Geometry: final body of the model. Coordinates: model frame, mm. A direction names the side the tool comes from. Round coordinates to 2 decimals unless told otherwise and drop trailing zeros. Loops run counter-clockwise (first coordinate to the right, second up) from the corner with the lowest first, then second, coordinate; pieces in that order, holes last. Notation, with made-up numbers: M -3.75,51 L 2.25,51 A28 ccw 2.25,83 Z; hole C -28.5,56 d7. An arc over 180 degrees is marked long. Answer as a JSON object with one key per item and string values.
from build123d import *

# Parameters (mm, degrees)
SKETCH1_W           = 60
SKETCH1_H           = 60
BOSS_EXTRUDE1_DEPTH = 100
SKETCH3_W           = 6
SKETCH3_H           = 12
CUT_EXTRUDE2_DEPTH  = 101


with BuildPart() as part:
    # Sketch1 → Boss-Extrude1 (new body)
    with BuildSketch(Plane.XY):
        with Locations((30, 30)):
            Rectangle(SKETCH1_W, SKETCH1_H)
    extrude(amount=-BOSS_EXTRUDE1_DEPTH)

    # Sketch3 → Cut-Extrude2 (cut, through all)
    with BuildSketch(Plane.XY):
        Polygon((26.781992624, 20), (33.218007376, 20), (50, 0), (10, 0), align=None)
        Polygon((26.781992624, 40), (33.218007376, 40), (50, 60), (10, 60), align=None)
        with Locations((57, 30)):
            Rectangle(SKETCH3_W, SKETCH3_H)
        with Locations((3, 30)):
            Rectangle(SKETCH3_W, SKETCH3_H)
    extrude(amount=-CUT_EXTRUDE2_DEPTH, mode=Mode.SUBTRACT)


solid = part.part
1) Section query D-D (y = 28.5). Return the cut outline in (x, z).
Results:
{"outline": "M 6,-100 L 54,-100 L 54,0 L 6,0 Z"}
2) Ray query, line 1 (Y direction, x = 54.5, z = -20); line 2 (Y direction, x = 29, z = -76); line 3 (X direction, y = 26, z = -21). Return the intervals inside material, ascending.
Results:
{"line 1": "0 to 24, 36 to 60", "line 2": "20 to 40", "line 3": "6 to 54"}
3) Section query A-A (x = 4). Return the cut outline in (y, z).
Results:
{"outline": "M 0,-100 L 24,-100 L 24,0 L 0,0 Z; M 36,-100 L 60,-100 L 60,0 L 36,0 Z"}
4) Pull-direction query (X, two-part tool) for faces 4 (the flat face through (30, 40, -49)), 5 (the flat face through (18.274, 9.86, -49.3)), 6 (the flat face through (6, 30, -49)), 7 (the flat face through (30, 30, -100)); classes: +X half, -X half, draft (parallel to the pull), parting line (faces both ways), or undercut.
Results:
{"face 4": "undercut", "face 5": "undercut", "face 6": "-X half", "face 7": "draft"}
5) Reachability of faces 1 (the flat face through (3, 36, -49)), 2 (the flat face through (30, 20, -49)), 3 (the flat face through (54, 30, -49)) from +Z, -Z, +X, -X, +Y, -Y: full face, straight path, thin tool, end or side. Return the list, or none.
Results:
{"face 1": "+Z, -Z, -X", "face 2": "+Z, -Z, -Y", "face 3": "+Z, -Z, +X"}
6) Section query B-B (y = 55). Return the cut outline in (x, z), and give its area (3 significant figures).
Results:
{"outline": "M 0,-100 L 14.2,-100 L 14.2,0 L 0,0 Z; M 45.8,-100 L 60,-100 L 60,0 L 45.8,0 Z", "area": "2,840 mm2"}
7) Pin query (flat end, axial travel): P1, Ø9.5, axis at y = 29.5, z = -68.5, coming from the +X side; P2, Ø12, axis at x = 21, z = -58, coming from the -Y side; P3, Ø1.9, axis at x = 30, z = -37, coming from the -Y side. Return the tip coordinate at first contact, or that it passes through.
Results:
{"P1": "x = 54", "P2": "y = 5.96", "P3": "y = 20"}
8) Section query C-C (z = -34.5). Return the cut outline in (x, y), and give its area (3 significant figures).
Results:
{"outline": "M 0,0 L 10,0 L 26.78,20 L 33.22,20 L 50,0 L 60,0 L 60,24 L 54,24 L 54,36 L 60,36 L 60,60 L 50,60 L 33.22,40 L 26.78,40 L 10,60 L 0,60 L 0,36 L 6,36 L 6,24 L 0,24 Z", "area": "2,530 mm2"}
